from build123d import *

# Parameters (mm, degrees)
SKETCH_2_R          = 2.25
CUT_EXTRUDE_1_DEPTH = 43.085211311


with BuildPart() as part:
    # ｽｹｯﾁ1 → 回転1 (revolve)
    with BuildSketch(Plane.XY, mode=Mode.PRIVATE) as revolve_1_sk:
        with BuildLine():
            Line((-25.75, 2), (-16.25, 2))
            Line((-16.25, 2), (-12.95, 5.3))
            Line((-12.95, 5.3), (-11.494781425, 5.3))
            ThreePointArc((-11.494781425, 5.3), (-6.808450631, 10.620774226), (0, 12.6))
            Line((0, 12.6), (0, -17.2))
            ThreePointArc((0, -17.2), (-11.532562595, -12.862446581), (-17.348198754, -2))
            Line((-17.348198754, -2), (-25.75, -2))
            ThreePointArc((-25.75, -2), (-27.75, 0), (-25.75, 2))
        make_face()
    revolve(revolve_1_sk.sketch.rotate(Axis((0, 0, 0), (0, -1, 0)), 270), axis=Axis((0, 0, 0), (0, -1, 0)))

    # ｽｹｯﾁ2 → ｶｯﾄ - 押し出し1 (cut, through all)
    with BuildSketch(Plane.XZ.offset(2)):
        with Locations(Location((-22.75, 0, 0), (0, 0, 270))):
            Circle(SKETCH_2_R)
        with Locations(Location((22.75, 0, 0), (0, 0, 90))):
            Circle(SKETCH_2_R)
    extrude(amount=-CUT_EXTRUDE_1_DEPTH, mode=Mode.SUBTRACT)


solid = part.part
Could you check a few things on this model? Use its own coordinates, in mm. A direction names the side the tool comes from. Round coordinates to 2 decimals unless told otherwise and drop trailing zeros. Loops run counter-clockwise (first coordinate to the right, second up) from the corner with the lowest first, then second, coordinate; pieces in that order, holes last. Notation, with made-up numbers: (5, 81) -> (48, 81) arc R5 cw to (48, 87) -> close; hole circle Ø2 at (18, 35). An arc over 180 degrees is marked (long way). Use CSV: the item, a comma, the result in double quotes.
(1) Suppose I cut it at A-A on z = 0. Write out the boundary of the cut face in (x, y).
Return value:
outline,"(-25.75, -2) -> (-25, -2) -> (-25, 2) -> (-25.75, 2) arc R2 ccw to start; (-20.5, -2) -> (-17.35, -2) arc R17.5 ccw to (17.35, -2) -> (20.5, -2) -> (20.5, 2) -> (16.25, 2) -> (12.95, 5.3) -> (11.49, 5.3) arc R12.7 ccw to (-11.49, 5.3) -> (-12.95, 5.3) -> (-16.25, 2) -> (-20.5, 2) -> close; (25, -2) -> (25.75, -2) arc R2 ccw to (25.75, 2) -> (25, 2) -> close"
(2) Will these pins go through, and if not, where does the flat tip stop? pin 1 Ø5 at (y, z) = (-4, -14) entering from +X; pin 2 Ø2 at (x, z) = (-22, 4) entering from +Y; pin 3 Ø3 at (y, z) = (7.5, 3) entering from +X; pin 4 Ø3.5 at (x, z) = (-22.75, 0) entering from +Y.
Return value:
pin 1,"stops at x = 23.45"
pin 2,"stops at y = 2"
pin 3,"stops at x = 10.81"
pin 4,"passes through"
(3) Suppose I cut it at C-C on y = -3.5. Write out the boundary of the cut face in (x, z).
Return value:
outline,"circle Ø34.16 at (0, 0)"
(4) Suppose I cut it at D-D on y = -11.25. Write out the boundary of the cut face in (x, z), plus the area to 3 significant figures.
Return value:
outline,"circle Ø26.29 at (0, 0)"
area,"543 mm²"
(5) If we mould it in two halves opening along X, with no side actions, what happens to faces 3 (the cylindrical face through (-25, 0, 0)), 4 (the conical face through (12.8, 5.14, -2.84)), 5 (the flat face through (17, -2, -5))? For each: +X half, -X half, draft (parallel to the pull), parting line (faces both ways), or undercut.
Return value:
face 3,"undercut"
face 4,"parting line"
face 5,"draft"
(6) If I drill on probe 1 along X at (y, z) = (0.6, 0); probe 2 along Y at (x, z) = (19, -9); probe 3 along Z at (x, y) = (22.75, 0), over which ranges is the centre line in solid material (lowest first)? Write a range as [from, to].
Return value:
probe 1,"x = [-27.66, -25], [-20.5, 20.5], [25, 27.66]"
probe 2,"y = [-2, 2]"
probe 3,"z = [-15.89, -2.25], [2.25, 15.89]"
(7) For faces 1 (the flat face through (17, 2, 0)), 2 (the cylindrical face through (25, 0, 0)), which set-ups out of +Z, -Z, +X, -X, +Y, -Y let a thin tool reach every point of the face, with its end or its side?
Return value:
face 1,"+Y"
face 2,"+Y, -Y"
(8) Suppose I cut it at B-B on x = 0. Write out the boundary of the cut face in (y, z), plus the area to 3 significant figures.
Return value:
outline,"(-2, -25.75) arc R2 ccw to (2, -25.75) -> (2, -16.25) -> (5.3, -12.95) -> (5.3, -11.49) arc R12.7 ccw to (5.3, 11.49) -> (5.3, 12.95) -> (2, 16.25) -> (2, 25.75) arc R2 ccw to (-2, 25.75) -> (-2, 17.35) arc R17.5 ccw to (-2, -17.35) -> close"
area,"836 mm²"
